Input: dimensioned drawing with shaded views. Units: mm. Origin: part minimum x, y, z. A direction names the side the tool comes from. Round coordinates to 2 decimals unless told otherwise and drop trailing zeros. Order: outer loops, then holes, each group sorted by start corner. A loop starts at its lowest first (then second) coordinate and runs counter-clockwise, first axis right, second up.
Item 1: Reachability of the marked faces 4 and 5 from +Z, -Z, +X, -X, +Y, -Y: full face, straight path, thin tool, end or side. Return the list, or none.
Item 2: Line query: L1, parallel to X at y = 5, z = 7; L2, parallel to Y at x = 4.5, z = 2.25. Output: solid intervals per line, ascending.
Item 3: Cut plane B-B on z = 12. Output: boundary loops of the cut face in (x, y).
Item 4: Cut plane D-D on z = 3.5. Output: boundary loops of the cut face in (x, y), then the cut area to 3 significant figures.
Item 5: Mould query, pull axis Y, two halves, no side actions, for the marked faces 1, 2 and 3. Classes: released by +Y, released by -Y, zero draft, split by the parting line, or undercut.
Item 6: Cut plane C-C on y = 6.5. Output: boundary loops of the cut face in (x, z).
Item 7: Cut plane A-A on x = 7. Output: boundary loops of the cut face in (y, z).
Item 8: First-contact query: pin 1 (5 mm diameter, centred on y = 4, z = 12.5, fed in from -X); pin 2 (2 mm diameter, centred on y = 1.5, z = 1.5, fed in from -X). Flat tips, straight axial feed; report the tip coordinate or a pass-through.
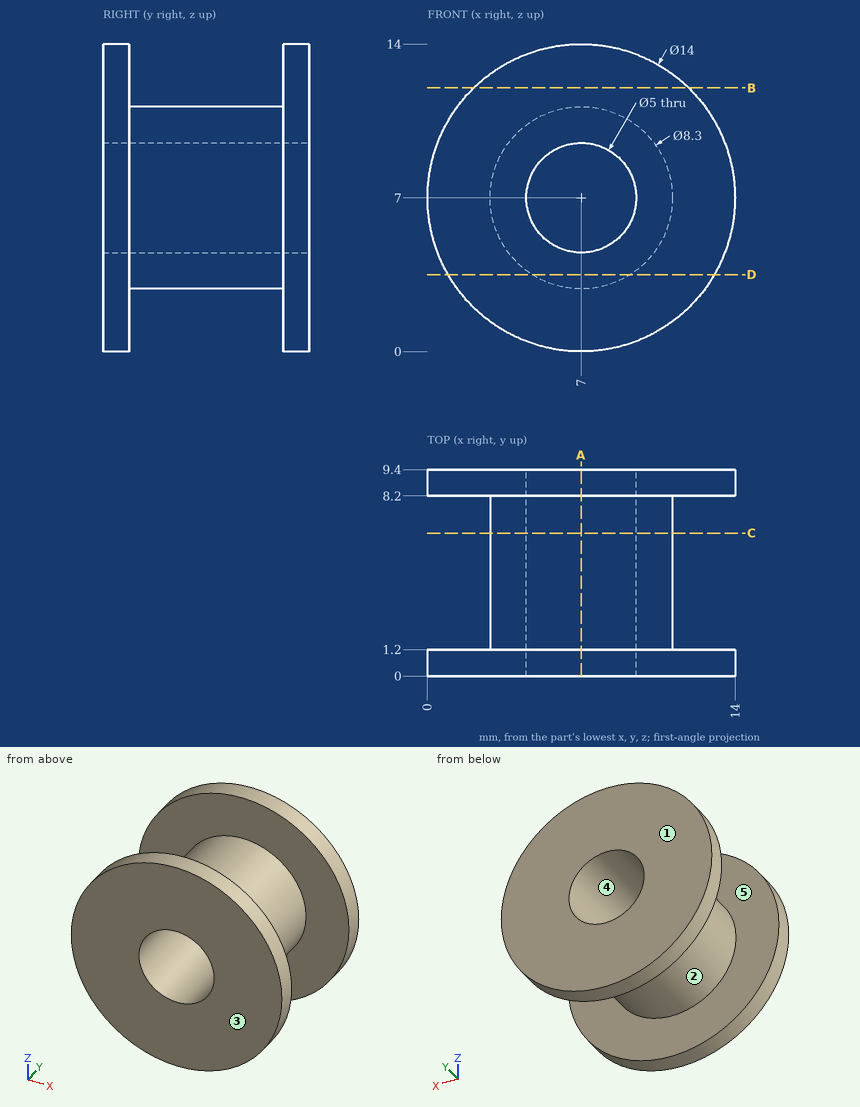
From the geometry:
1. face 4: +Y, -Y
1. face 5: none
2. L1: x = 2.85 to 4.5, 9.5 to 11.15
2. L2: y = 0 to 1.2, 8.2 to 9.4
3. outline: (2.1, 0) - (11.9, 0) - (11.9, 1.2) - (2.1, 1.2) - close; (2.1, 8.2) - (11.9, 8.2) - (11.9, 9.4) - (2.1, 9.4) - close
4. outline: (0.94, 0) - (13.06, 0) - (13.06, 1.2) - (9.23, 1.2) - (9.23, 8.2) - (13.06, 8.2) - (13.06, 9.4) - (0.94, 9.4) - (0.94, 8.2) - (4.77, 8.2) - (4.77, 1.2) - (0.94, 1.2) - close
4. area: 60.3 mm2
5. face 1: released by +Y
5. face 2: undercut
5. face 3: released by -Y
6. outline: circle Ø8.3 at (7, 7); hole circle Ø5 at (7, 7)
7. outline: (0, 0) - (1.2, 0) - (1.2, 2.85) - (8.2, 2.85) - (8.2, 0) - (9.4, 0) - (9.4, 4.5) - (0, 4.5) - close; (0, 9.5) - (9.4, 9.5) - (9.4, 14) - (8.2, 14) - (8.2, 11.15) - (1.2, 11.15) - (1.2, 14) - (0, 14) - close
8. pin 1: stops at x = 4.13
8. pin 2: stops at x = 1.68
